from build123d import *

# Parameters (mm, degrees)
SKETCH_1_R      = 1.5
SKETCH_1_W      = 21
SKETCH_1_H      = 42
EXTRUDE_1_DEPTH = 3


with BuildPart() as part:
    # 草圖1 → 填料-伸長1 (new body)
    with BuildSketch(Plane(origin=(0, 0, 0), x_dir=(1, 0, 0), z_dir=(0, 1, 0))):
        Polygon((11.5, 22), (11.5, -22), (11.5, -26), (-11.5, -26), (-11.5, -22), (-11.5, 22), (-11.5, 26), (11.5, 26), align=None)
        with Locations((-4.7, 23.8)):
            Circle(SKETCH_1_R, mode=Mode.SUBTRACT)
        with Locations((4.7, 23.8)):
            Circle(SKETCH_1_R, mode=Mode.SUBTRACT)
        with Locations((4.7, -23.8)):
            Circle(SKETCH_1_R, mode=Mode.SUBTRACT)
        with Locations((-4.7, -23.8)):
            Circle(SKETCH_1_R, mode=Mode.SUBTRACT)
        Rectangle(SKETCH_1_W, SKETCH_1_H, mode=Mode.SUBTRACT)
    extrude(amount=EXTRUDE_1_DEPTH)


solid = part.part
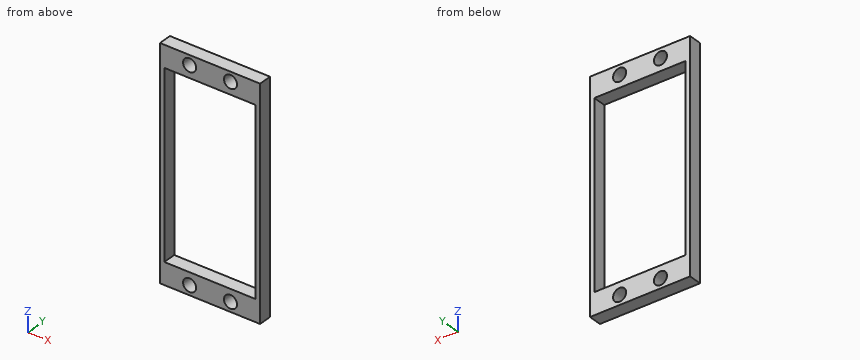
Geometry: final body of the model. Coordinates: model frame, mm. Give positions to 0.01 mm unless a question says otherwise; leave off trailing zeros. Write each loop counter-clockwise with the first axis right and the second up, starting at its lowest first coordinate (ties: lowest second). Pieces come first, ordered by that corner, then holes. Notation, with made-up numbers: (-32.75, 52) -> (15.25, 52) arc R16 ccw to (15.25, 68) -> close; hole circle Ø8 at (-5, 64.25). An arc over 180 degrees is marked (long way). Answer in a Markdown table with one row per item.
(1) Section query B-B on z = -23.8. Return loops of the section in (x, y).
Answers below:
| item | result |
|---|---|
| outline | (-11.5, 0) -> (-6.2, 0) -> (-6.2, 3) -> (-11.5, 3) -> close; (-3.2, 0) -> (3.2, 0) -> (3.2, 3) -> (-3.2, 3) -> close; (6.2, 0) -> (11.5, 0) -> (11.5, 3) -> (6.2, 3) -> close |
(2) Section query C-C on y = 1.6. Return loops of the section in (x, z), then the cut area to 3 significant figures.
Answers below:
| item | result |
|---|---|
| outline | (-11.5, -26) -> (11.5, -26) -> (11.5, 26) -> (-11.5, 26) -> close; hole (-10.5, -21) -> (10.5, -21) -> (10.5, 21) -> (-10.5, 21) -> close; hole circle Ø3 at (-4.7, -23.8); hole circle Ø3 at (-4.7, 23.8); hole circle Ø3 at (4.7, -23.8); hole circle Ø3 at (4.7, 23.8) |
| area | 286 mm^2 |
(3) Section query A-A on x = 4.7. Return loops of the section in (y, z), then the cut area to 3 significant figures.
Answers below:
| item | result |
|---|---|
| outline | (0, -26) -> (3, -26) -> (3, -25.3) -> (0, -25.3) -> close; (0, -22.3) -> (3, -22.3) -> (3, -21) -> (0, -21) -> close; (0, 21) -> (3, 21) -> (3, 22.3) -> (0, 22.3) -> close; (0, 25.3) -> (3, 25.3) -> (3, 26) -> (0, 26) -> close |
| area | 12.0 mm^2 |
(4) Section query D-D on x = -7.75. Return loops of the section in (y, z).
Answers below:
| item | result |
|---|---|
| outline | (0, -26) -> (3, -26) -> (3, -21) -> (0, -21) -> close; (0, 21) -> (3, 21) -> (3, 26) -> (0, 26) -> close |
(5) Ray query, line 1 along Z through (x, y) = (-4.7, 0.7); line 2 along X through (y, z) = (2.15, 23.8); line 3 along X through (y, z) = (1.85, -10). Return the intervals inside material, ascending. Write a range as [from, to].
Answers below:
| item | result |
|---|---|
| line 1 | [-26, -25.3], [-22.3, -21], [21, 22.3], [25.3, 26] |
| line 2 | [-11.5, -6.2], [-3.2, 3.2], [6.2, 11.5] |
| line 3 | [-11.5, -10.5], [10.5, 11.5] |
(6) Pin query (flat end, axial travel): pin 1 (2.5 mm diameter, centred on x = 4.7, z = -23.8, fed in from -Y). Return the tip coordinate at first contact, or that it passes through.
Answers below:
| item | result |
|---|---|
| pin 1 | through |
